```python
from build123d import *

# Parameters (mm, degrees)
BOSS_EXTRUDE1_DEPTH      = 25.4
BOSS_EXTRUDE1_DEPTH_BACK = 50.8
SKETCH1_R                = 38.1
SKETCH1_3_R              = 50.8
SKETCH1_3_R_2            = 38.1
BOSS_EXTRUDE2_DEPTH      = 6.35


with BuildPart() as part:
    # Sketch1 → Boss-Extrude1 (new, two sides: drawn at the far end of the back side and taken through both)
    with BuildSketch(Plane(origin=(0, 0, 0), x_dir=(1, 0, 0), z_dir=(0, 1, 0)).offset(-BOSS_EXTRUDE1_DEPTH_BACK)):
        with Locations(Location((0, 0, 0), (0, 0, 270))):
            Circle(SKETCH1_R)
    extrude(amount=BOSS_EXTRUDE1_DEPTH + BOSS_EXTRUDE1_DEPTH_BACK)

    # Sketch1_3 → Boss-Extrude2 (add)
    with BuildSketch(Plane(origin=(0, 0, 0), x_dir=(1, 0, 0), z_dir=(0, 1, 0))):
        with Locations(Location((0, 0, 0), (0, 0, 270))):
            Circle(SKETCH1_3_R)
        with Locations(Location((0, 0, 0), (0, 0, 270))):
            Circle(SKETCH1_3_R_2, mode=Mode.SUBTRACT)
    extrude(amount=BOSS_EXTRUDE2_DEPTH)


solid = part.part
```
Could you check a few things on this model? Use its own coordinates, in mm. A direction names the side the tool comes from. Give positions to 0.01 mm unless a question says otherwise; leave off trailing zeros. Loops run counter-clockwise (first coordinate to the right, second up) from the corner with the lowest first, then second, coordinate; pieces in that order, holes last. Notation, with made-up numbers: (45, 47) -> (81, 47) arc R18 ccw to (81, 80) -> close; hole circle Ø4 at (9.5, 15.5). An arc over 180 degrees is marked (long way). Put each result on its own line as item: value.
(1) For faces 1 (the face through (-23.183, 15.742, -30.235)), 2 (the face through (38, 0, 7)), 3 (the face through (1, -50.8, -1)), which set-ups out of +Z, -Z, +X, -X, +Y, -Y let a thin tool reach every point of the face, with its end or its side?
Computed:
face 1: +Y
face 2: -Y
face 3: +Z, -Z, +X, -X, -Y
(2) Imagine slicing it at B-B on z = 0. Write out the boundary of the cut face in (x, y), plus the area to 3 significant figures.
Computed:
outline: (-50.8, 0) -> (-38.1, 0) -> (-38.1, -50.8) -> (38.1, -50.8) -> (38.1, 0) -> (50.8, 0) -> (50.8, 6.35) -> (38.1, 6.35) -> (38.1, 25.4) -> (-38.1, 25.4) -> (-38.1, 6.35) -> (-50.8, 6.35) -> close
area: 5,970 mm^2
(3) Please list where these lines run through material, in increasing order: probe 1 along Y at (x, z) = (4, 45.5); probe 2 along Z at (x, y) = (-1.5, -26); probe 3 along Z at (x, y) = (29, 19). Write a range as [from, to].
Computed:
probe 1: [0, 6.35]
probe 2: [-38.07, 38.07]
probe 3: [-24.71, 24.71]
(4) Imagine slicing it at D-D on z = 40.5. Write out the boundary of the cut face in (x, y).
Computed:
outline: (-30.67, 0) -> (30.67, 0) -> (30.67, 6.35) -> (-30.67, 6.35) -> close
(5) I'm going to push flat-ended pins straight in: pin 1 Ø10 at (y, z) = (5, -19.5) entering from -X; pin 2 Ø12 at (y, z) = (-24.5, -39) entering from +X; pin 3 Ø4 at (x, z) = (22, -34) entering from +Y. Where does each tip first touch, or does it pass through?
Computed:
pin 1: x = -48.69
pin 2: x = 19.04
pin 3: y = 6.35
(6) Imagine slicing it at A-A on x = 0. Write out the boundary of the cut face in (y, z).
Computed:
outline: (-50.8, -38.1) -> (0, -38.1) -> (0, -50.8) -> (6.35, -50.8) -> (6.35, -38.1) -> (25.4, -38.1) -> (25.4, 38.1) -> (6.35, 38.1) -> (6.35, 50.8) -> (0, 50.8) -> (0, 38.1) -> (-50.8, 38.1) -> close
(7) Imagine slicing it at C-C on y = 15.5. Write out the boundary of the cut face in (x, z), plus the area to 3 significant figures.
Computed:
outline: circle Ø76.2 at (0, 0)
area: 4,560 mm^2
